Check sheet for the drawn part. Datum: minimum x, y, z corner. Units: mm. A direction names the side the tool comes from. Round coordinates to 2 decimals unless told otherwise and drop trailing zeros. Order: outer loops, then holes, each group sorted by start corner. A loop starts at its lowest first (then second) coordinate and runs counter-clockwise, first axis right, second up. Notation, with made-up numbers: (36.5, 12.25) -> (67.5, 12.25) arc R25 ccw to (67.5, 26.25) -> close; hole circle Ø5 at (54.5, 40.25). An arc over 180 degrees is marked (long way). Answer in a Markdown table with one row per item.
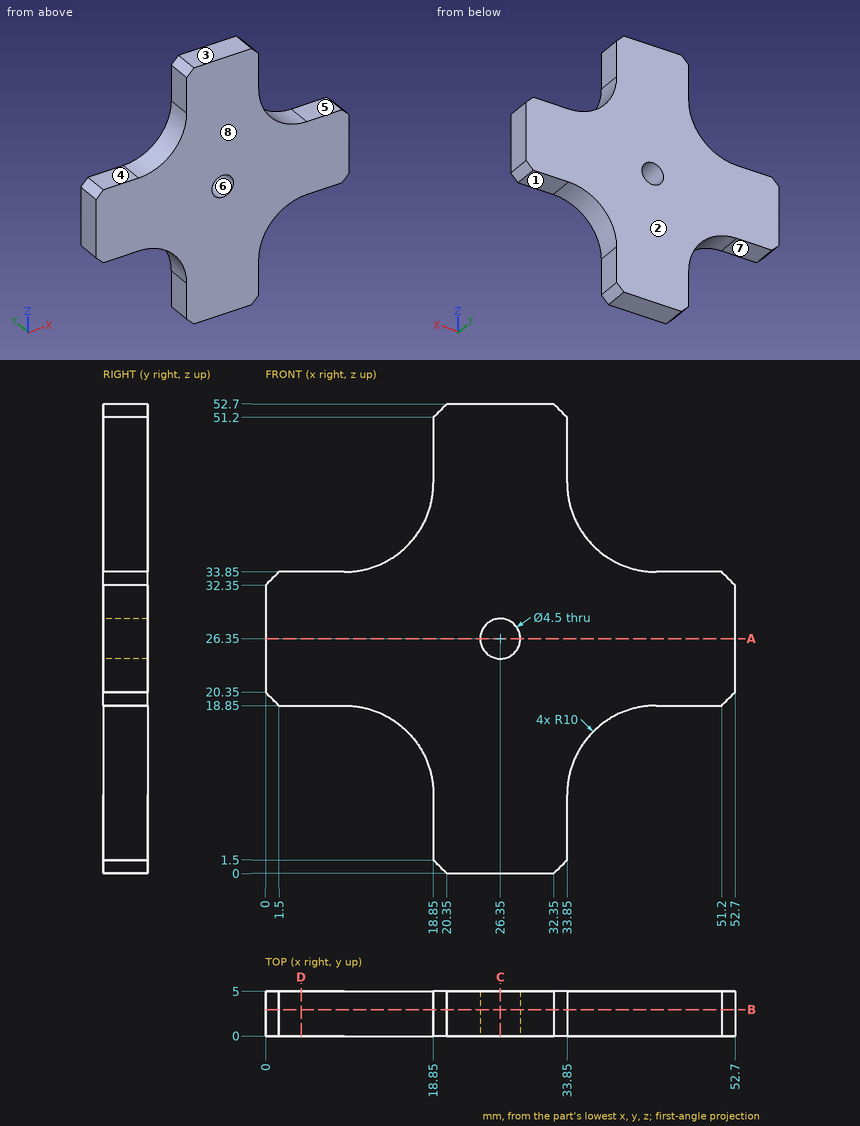
(1) Section check A-A on z = 26.35. Record the boundary of the cut face in (x, y).
Solutions:
| item | result |
|---|---|
| outline | (0, 0) -> (24.1, 0) -> (24.1, 5) -> (0, 5) -> close; (28.6, 0) -> (52.7, 0) -> (52.7, 5) -> (28.6, 5) -> close |
(2) Depth check by flat-ended pin: pin 1 Ø2.5 at (x, y) = (3.5, 3.5) entering from -Z; pin 2 Ø1.5 at (y, z) = (3, 49) entering from +X; pin 3 Ø1.5 at (x, y) = (6, 2.5) entering from +Z. Enter the tip coordinate at first touch or a pass-through.
Solutions:
| item | result |
|---|---|
| pin 1 | z = 18.85 |
| pin 2 | x = 33.85 |
| pin 3 | z = 33.85 |
(3) Section check C-C on x = 26.35. Record the boundary of the cut face in (y, z).
Solutions:
| item | result |
|---|---|
| outline | (0, 0) -> (5, 0) -> (5, 24.1) -> (0, 24.1) -> close; (0, 28.6) -> (5, 28.6) -> (5, 52.7) -> (0, 52.7) -> close |
(4) Section check B-B on y = 2.95. Record the boundary of the cut face in (x, z).
Solutions:
| item | result |
|---|---|
| outline | (0, 20.35) -> (1.5, 18.85) -> (8.85, 18.85) arc R10 cw to (18.85, 8.85) -> (18.85, 1.5) -> (20.35, 0) -> (32.35, 0) -> (33.85, 1.5) -> (33.85, 8.85) arc R10 cw to (43.85, 18.85) -> (51.2, 18.85) -> (52.7, 20.35) -> (52.7, 32.35) -> (51.2, 33.85) -> (43.85, 33.85) arc R10 cw to (33.85, 43.85) -> (33.85, 51.2) -> (32.35, 52.7) -> (20.35, 52.7) -> (18.85, 51.2) -> (18.85, 43.85) arc R10 cw to (8.85, 33.85) -> (1.5, 33.85) -> (0, 32.35) -> close; hole circle Ø4.5 at (26.35, 26.35) |
(5) Scan lines: probe 1 along X at (y, z) = (1.75, 26.35); probe 2 along Z at (x, y) = (2, 3.1). Record each from-to range of solid material in increasing order. Write a range as from..to.
Solutions:
| item | result |
|---|---|
| probe 1 | 0..24.1, 28.6..52.7 |
| probe 2 | 18.85..33.85 |
(6) Section check D-D on x = 4. Record the boundary of the cut face in (y, z), plus the area to 3 significant figures.
Solutions:
| item | result |
|---|---|
| outline | (0, 18.85) -> (5, 18.85) -> (5, 33.85) -> (0, 33.85) -> close |
| area | 75.0 mm^2 |
(7) Tool access check on the marked faces 1, 2, 3, 4 and 5. Record the directions out of +Z, -Z, +X, -X, +Y, -Y that give a thin tool (end or side, any length) a straight path to the whole face; none if there is none.
Solutions:
| item | result |
|---|---|
| face 1 | -Z, +X, +Y, -Y |
| face 2 | +Z, -Z, +X, -X, +Y |
| face 3 | +Z, +X, -X, +Y, -Y |
| face 4 | +Z, -X, +Y, -Y |
| face 5 | +Z, +X, +Y, -Y |
(8) Draft check along Z on the marked faces 6, 7 and 8. Enter one of: pulls with the +Z half, pulls with the -Z half, needs draft (parallel to the pull), parting line crosses it, or undercut.
Solutions:
| item | result |
|---|---|
| face 6 | undercut |
| face 7 | pulls with the -Z half |
| face 8 | needs draft |
